Here's how the part is built. I have some questions about the finished solid (model axes, mm). A direction names the side the tool comes from. Coordinates: 2 decimals unless noted, no trailing zeros. Write each loop counter-clockwise with the first axis right and the second up, starting at its lowest first coordinate (ties: lowest second). Pieces come first, ordered by that corner, then holes.
Item 1: If we section it at D-D (x = -27): Please give me the cut outline in (y, z) (3 decimals), then the cut area to 3 significant figures.
Item 2: If we section it at C-C (x = 3): Please give me the cut outline in (y, z) (1 decimal).
Item 3: For faces 1 (the face through (-0.178, -4.336, -19.524)), 2 (the face through (11.46, 10.6, 3.34)), 3 (the face through (0, -11, -3)), which set-ups out of +Z, -Z, +X, -X, +Y, -Y let a thin tool reach every point of the face, with its end or its side?
Item 4: We'd pull the mould along X, two halves only. Please class faces 4 (the face through (-15.466, -3.441, -15.497)), 5 (the face through (-12.7, -13, -16)), 6 (the face through (22.612, -11, -5)): +X half, -X half, draft (parallel to the pull), parting line (faces both ways), or undercut.
Item 5: I'm going to push flat-ended pins straight in: pin 1 Ø6 at (x, y) = (-22, -15) entering from +Z; pin 2 Ø5 at (x, y) = (-16.5, -10) entering from -Z; pin 3 Ø6 at (x, z) = (-0.5, 17) entering from +Y. Where does each tip first touch, or does it pass through?
Item 6: If I drill on line 1 (Z direction, x = 11.75, y = 0); line 2 (Z direction, x = -2, y = 9); line 3 (Y direction, x = -3, z = 11), over which ranges is the centre line in solid material (lowest first)?
from build123d import *

# Parameters (mm, degrees)
FILLET1_R = 1.27


with BuildPart() as part:
    # Sketch1 → Revolve1 (revolve)
    with BuildSketch(Plane.XY):
        Polygon((0, 11.1125), (22.612386478, 11.1125), (22.612386478, 25.4), (21.024886478, 25.4), (19.558416794, 22.86), (12.7, 22.86), (12.7, 20), (-12.7, 20), (-12.7, 22.86), (-31.370233522, 19.05), (-31.370233522, 15.875), (0, 15.875), align=None)
    revolve(axis=Axis((-42.201018363, 0, 0), (1, 0, 0)))

    # Fillet1
    fillet1_edges = [part.edges().sort_by_distance(p)[0] for p in [
        (12.7, -22.86, 0),
        (-31.370233522, -19.05, 0),
        (-12.7, -22.86, 0),
    ]]
    fillet(fillet1_edges, radius=FILLET1_R)


solid = part.part
Answer list:
1. outline: circle Ø39.884 at (0, 0); hole circle Ø31.75 at (0, 0)
1. area: 458 mm2
2. outline: circle Ø40 at (0, 0); hole circle Ø22.2 at (0, 0)
3. face 1: none
3. face 2: +X, -X
3. face 3: -X
4. face 4: draft
4. face 5: undercut
4. face 6: +X half
5. pin 1: stops at z = 17.32
5. pin 2: stops at z = -20.92
5. pin 3: stops at y = 14.28
6. line 1: z = -20 to -11.11, 11.11 to 20
6. line 2: z = -17.86 to -13.08, 13.08 to 17.86
6. line 3: y = -16.7 to -11.45, 11.45 to 16.7
